Build history of the part. All positions in model axes, mm. A direction names the side the tool comes from. Give positions to 0.01 mm unless a question says otherwise; leave off trailing zeros. Order: outer loops, then holes, each group sorted by start corner. A loop starts at its lowest first (then second) coordinate and runs counter-clockwise, first axis right, second up. Notation, with made-up numbers: (-20.75, 56) - (-5.75, 56) arc R24 ccw to (-5.75, 89) - close; hole circle Ø3 at (44.25, 75.25). An arc over 180 degrees is marked (long way). Use a Markdown table: item, result.
from build123d import *

# Parameters (mm, degrees)
F1_DEPTH = 25.4
F2_R     = 3.175
F3_DEPTH = 25.4
F4_T     = -2.54


with BuildPart() as f1:
    # F0 (on Front) → F1 (new body)
    with BuildSketch(Plane.XZ):
        with BuildLine():
            ThreePointArc((24.638, 0), (17.4216968749, 17.4216968749), (0, 24.638))
            ThreePointArc((0, 24.638), (-17.4216968749, 17.4216968749), (-24.638, 0))
            Line((-24.638, 0), (-12.7, -21.0615165602))
            Line((-12.7, -21.0615165602), (0, 0))
            Line((0, 0), (12.7, -21.0615165602))
            Line((12.7, -21.0615165602), (24.638, 0))
        make_face()
    extrude(amount=F1_DEPTH)

    # F2 (on face) → F3 (join)
    with BuildSketch(Plane.XZ.offset(25.4)):
        with Locations((0, 7.7885312092)):
            Circle(F2_R)
    extrude(amount=F3_DEPTH)

    # F4
    f4_openings = [f1.faces().sort_by_distance(p)[0] for p in [
        (0, -50.8, 7.788531),
    ]]
    offset(amount=F4_T, openings=f4_openings, kind=Kind.INTERSECTION)


solid = f1.part
1) Slice it at D-D (x = -15.5). Write the cut outline in (y, z), and give its area (3 significant figures).
Computed:
| item | result |
|---|---|
| outline | (-25.4, -16.12) - (0, -16.12) - (0, 19.15) - (-25.4, 19.15) - close; hole (-22.86, -10.97) - (-2.54, -10.97) - (-2.54, 15.75) - (-22.86, 15.75) - close |
| area | 353 mm² |
2) Two-plate mould, pull along Y, no slides. Class faces 5 (the flat face through (-18.753, -12.522, -10.383)), 6 (the flat face through (-6.405, -12.558, -5.702)), 7 (the flat face through (0, 0, 2)), 8 (the flat face through (0, -25.4, 2)): +Y half, -Y half, draft (parallel to the pull), parting line (faces both ways), or undercut.
Computed:
| item | result |
|---|---|
| face 5 | draft |
| face 6 | undercut |
| face 7 | +Y half |
| face 8 | -Y half |
3) Slice it at A-A (z = -18). Write the cut outline in (x, y), and give its area (3 significant figures).
Computed:
| item | result |
|---|---|
| outline | (-14.44, -25.4) - (-10.85, -25.4) - (-10.85, 0) - (-14.44, 0) - close; (10.85, -25.4) - (14.44, -25.4) - (14.44, 0) - (10.85, 0) - close |
| area | 182 mm² |
4) Slice it at B-B (x = 20). Write the cut outline in (y, z).
Computed:
| item | result |
|---|---|
| outline | (-25.4, -8.18) - (0, -8.18) - (0, 14.39) - (-25.4, 14.39) - close; hole (-22.86, -3.03) - (-2.54, -3.03) - (-2.54, 9.4) - (-22.86, 9.4) - close |
5) Pin check, flat tips, straight feed: P1, Ø8, axis at x = -0.5, y = -11, coming from the -Z side; P2, Ø1.5, axis at x = 11.5, y = -9.5, coming from the +Z side; P3, Ø6, axis at x = 0.5, y = -23, coming from the -Z side; P4, Ø8, axis at y = -45.5, z = 15, coming from the +X side (1 decimal). Stop position of each tip, or through.
Computed:
| item | result |
|---|---|
| P1 | stops at z = -7.46 |
| P2 | stops at z = 22.17 |
| P3 | stops at z = -5.8 |
| P4 | passes through |
6) Tool access for faces 1 (the flat face through (-5, -22.86, 8)), 2 (the cylindrical face through (-0.08, -36.63, 8.42)), 3 (the flat face through (1, -50.8, 8)), 4 (the flat face through (6.26, -12.52, -10.38)): list every direction of +Z, -Z, +X, -X, +Y, -Y with a clear straight run to the whole face (end or side of a thin tool).
Computed:
| item | result |
|---|---|
| face 1 | none |
| face 2 | -Y |
| face 3 | +Z, -Z, +X, -X, -Y |
| face 4 | -Z, +Y, -Y |
7) Wall check: line 1 (Z direction, x = 0, y = -42); line 2 (X direction, y = -14, z = -14); line 3 (Y direction, x = 6, z = 9.5). Give the ranges that are in metal, low to high. Write a range as from..to.
Computed:
| item | result |
|---|---|
| line 1 | z = 4.61..7.15, 8.42..10.96 |
| line 2 | x = -16.7..-13.78, -11.41..-8.44, 8.44..11.41, 13.78..16.7 |
| line 3 | y = -25.4..-22.86, -2.54..0 |
8) Slice it at C-C (y = -14.5). Write the cut outline in (x, z), and give its area (3 significant figures).
Computed:
| item | result |
|---|---|
| outline | (-24.64, 0) - (-12.7, -21.06) - (0, 0) - (12.7, -21.06) - (24.64, 0) arc R24.64 ccw to start; hole (-22.09, 0.65) - (-12.63, -16.03) - (0, 4.92) - (12.63, -16.03) - (22.09, 0.65) arc R22.1 ccw to start |
| area | 420 mm² |
